```python
from build123d import *

# Parameters (mm, degrees)
F0_R     = 9
F0_R_2   = 1.4
F1_DEPTH = 3


with BuildPart() as f1:
    # F0 (on Top) → F1 (new body)
    with BuildSketch(Plane.XY):
        with Locations((-25.063416, 15.770752)):
            Circle(F0_R)
        with Locations((-25.063416, 15.770752)):
            Circle(F0_R_2, mode=Mode.SUBTRACT)
    extrude(amount=F1_DEPTH)


with BuildPart() as f1_1:
    # F3: moved
    add(f1.part.moved(Location((25.1714, 0, 0))))


with BuildPart() as f1_2:
    # F4: moved
    add(f1_1.part.moved(Location((-0.10792, -15.77066, 0))))

    # F2 (on Right) → F6 (revolve, cut)
    with BuildSketch(Plane.YZ):
        with BuildLine():
            ThreePointArc((-8.092892, 0.83043), (-7.67323, 1.008644), (-7.5, 1.430388))
            ThreePointArc((-7.5, 1.430388), (-7.678471, 1.857369), (-8.10771, 2.030338))
            ThreePointArc((-8.10771, 2.030338), (-8.699954, 1.422979), (-8.092892, 0.83043))
        make_face()
        with BuildLine():
            ThreePointArc((-8.092892, 0.83043), (-8.699954, 1.422979), (-8.10771, 2.030338))
            Line((-8.10771, 2.030338), (-10.503868, 2.030338))
            Line((-10.503868, 2.030338), (-10.503868, 0.801864))
            Line((-10.503868, 0.801864), (-8.092892, 0.83043))
        make_face()
    revolve(axis=Axis((0, 0, 1.962848), (0, 0, -1)), mode=Mode.SUBTRACT)


solid = f1_2.part
```
Here's how the part is built. I have some questions about the finished solid (model axes, mm). Coordinates: 2 decimals unless noted, no trailing zeros. Write each loop counter-clockwise with the first axis right and the second up, starting at its lowest first coordinate (ties: lowest second). Pieces come first, ordered by that corner, then holes. Notation, with made-up numbers: (13.25, 13) -> (24.25, 13) arc R8 cw to (24.25, 17) -> close; hole circle Ø5 at (18.5, 31.5). An arc over 180 degrees is marked (long way). Use a Markdown table: item, result. Add a question column.
(1) If we section it at B-B, the plane z = 1.05: Write out the boundary of the cut face in (x, y).
(2) I'm going to push a flat-ended pin straight in: P1, Ø1.7, axis at x = 0, y = 0, coming from the +Z side. Where does the tip first touch, or does it pass through?
(3) If we section it at A-A, the plane x = 0: Write out the boundary of the cut face in (y, z), and give its area (3 significant figures).
(4) Please list where these lines run through material, in increasing order: line 1 (Z direction, x = -8, y = 4); line 2 (X direction, y = 0.25, z = 2.9); line 3 (Y direction, x = 1, z = 2.8).
(5) We'd pull the mould along Z, two halves only. Please class faces 1 (the flat face through (2, 0, 0)), 2 (the flat face through (-5, -7, 2.03)), 3 (the cylindrical face through (8.584, 2.703, 2.508)): +Z half, -Z half, draft (parallel to the pull), parting line (faces both ways), or undercut.
Outcome:
| question | item | result |
|---|---|---|
| 1 | outline | circle Ø15.27 at (0, 0); hole circle Ø2.8 at (0, 0) |
| 2 | P1 | passes through |
| 3 | outline | (-9, 0) -> (-1.4, 0) -> (-1.4, 3) -> (-9, 3) -> (-9, 2.03) -> (-8.11, 2.03) arc R0.6 cw to (-7.5, 1.43) arc R0.6 cw to (-8.09, 0.83) -> (-9, 0.82) -> close; (1.4, 0) -> (9, 0) -> (9, 0.82) -> (8.09, 0.83) arc R0.6 cw to (7.5, 1.43) arc R0.6 cw to (8.11, 2.03) -> (9, 2.03) -> (9, 3) -> (1.4, 3) -> close |
| 3 | area | 42.3 mm^2 |
| 4 | line 1 | z = 0 to 0.82, 2.03 to 3 |
| 4 | line 2 | x = -9 to -1.38, 1.38 to 9 |
| 4 | line 3 | y = -8.94 to -0.98, 0.98 to 8.94 |
| 5 | face 1 | -Z half |
| 5 | face 2 | undercut |
| 5 | face 3 | draft |
